Design review of the part built by this model. Coordinates are the model's own, in mm. Face numbers are marked on the shaded views. A direction names the side the tool comes from. Coordinates: 2 decimals unless noted, no trailing zeros. Order: outer loops, then holes, each group sorted by start corner. A loop starts at its lowest first (then second) coordinate and runs counter-clockwise, first axis right, second up. Notation, with made-up numbers: M 20.25,19 L 33.25,19 A18 cw 33.25,31 Z; hole C 48.5,-37.5 d7. An arc over 180 degrees is marked long. Answer in a Markdown table with one row per item.
from build123d import *

# Parameters (mm, degrees)
F3_D     = 3
F3_DEPTH = 5
F3_TIP   = 0.9012909285
F4_DEPTH = 3


with BuildPart() as f1:
    # F0 (on Front) → F1 (revolve)
    with BuildSketch(Plane.XZ):
        Polygon((-8, 4.25), (-8, 0), (25, 0), (25, 2.5), (0, 2.5), (0, 4.25), align=None)
    revolve(axis=Axis((8.5, 0, 0), (-1, 0, 0)))

    # F3
    with Locations(Plane(origin=(-8, 0, 0), x_dir=(0, -1, 0), z_dir=(-1, 0, 0))):
        with Locations((0, 0)):
            Hole(F3_D / 2, depth=F3_DEPTH)
            with Locations((0, 0, -(F3_DEPTH + F3_TIP / 2))):  # 118° drill point
                Cone(0, F3_D / 2, F3_TIP, mode=Mode.SUBTRACT)

    # F2 (on face) → F4 (cut)
    with BuildSketch(Plane(origin=(-8, 0, 0), x_dir=(0, -1, 0), z_dir=(-1, 0, 0))):
        Polygon((-1.1547005384, -2), (1.1547005384, -2), (2.3094010768, 0), (1.1547005384, 2), (-1.1547005384, 2), (-2.3094010768, 0), align=None)
    extrude(amount=-F4_DEPTH, mode=Mode.SUBTRACT)


solid = f1.part
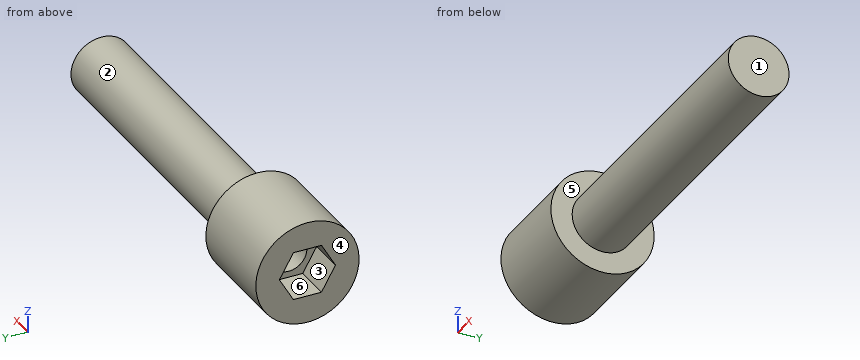
(1) Draft analysis for pull direction Y (two halves, no side actions). For the marked faces 1, 2 and 3, state which applies: pulls with the +Y half, pulls with the -Y half, needs draft (parallel to the pull), parting line crosses it, or undercut.
Return value:
| item | result |
|---|---|
| face 1 | needs draft |
| face 2 | parting line crosses it |
| face 3 | undercut |
(2) Insertion check: pin 1 Ø5 at (x, z) = (6.5, 1) entering from +Y; pin 2 Ø2.5 at (y, z) = (0, 0) entering from -X; pin 3 Ø1 at (x, y) = (-3.5, -3) entering from -Z. Each pin has a flat end and moves straight along its axis. Give the tip position at first contact, or say it passes through.
Return value:
| item | result |
|---|---|
| pin 1 | stops at y = 2.5 |
| pin 2 | stops at x = -2.85 |
| pin 3 | stops at z = -3.44 |
(3) Add section A-A, the plane x = -4.5. Give the boundary of the cut face in (y, z).
Return value:
| item | result |
|---|---|
| outline | C 0,0 d8.5; hole C 0,0 d3 |
(4) For the marked faces 4, 5 and 6, list the 3-axis set-ups (+Z, -Z, +X, -X, +Y, -Y) from which the entire face can be reached by the end or side of a thin tool; tool diameter is ignored.
Return value:
| item | result |
|---|---|
| face 4 | +Z, -Z, -X, +Y, -Y |
| face 5 | +X |
| face 6 | -X |
(5) Add section B-B, the plane x = 4. Give the boundary of the cut face in (y, z), and give its area (3 significant figures).
Return value:
| item | result |
|---|---|
| outline | C 0,0 d5 |
| area | 19.6 mm2 |
(6) For line 1 along Y through (x, z) = (-4.35, 0); line 2 along X through (y, z) = (4, 0.75); line 3 along Y through (x, z) = (-4.5, -1), list the stretches that pass through material, from the lowest coordinate up. Write a range as from..to.
Return value:
| item | result |
|---|---|
| line 1 | y = -4.25..-1.5, 1.5..4.25 |
| line 2 | x = -8..0 |
| line 3 | y = -4.13..-1.12, 1.12..4.13 |
(7) Add section C-C, the plane z = -3.25. Give the boundary of the cut face in (x, y).
Return value:
| item | result |
|---|---|
| outline | M -8,-2.74 L 0,-2.74 L 0,2.74 L -8,2.74 Z |
(8) Add section D-D, the plane y = 3.5. Give the boundary of the cut face in (x, z).
Return value:
| item | result |
|---|---|
| outline | M -8,-2.41 L 0,-2.41 L 0,2.41 L -8,2.41 Z |
